Design review of the part built by this model. Coordinates are the model's own, in mm. Face numbers are marked on the shaded views. A direction names the side the tool comes from. Round coordinates to 2 decimals unless told otherwise and drop trailing zeros. Order: outer loops, then holes, each group sorted by start corner. A loop starts at its lowest first (then second) coordinate and runs counter-clockwise, first axis right, second up. Notation, with made-up numbers: M 46.25,88.5 L 91.25,88.5 A23 cw 91.25,98.5 Z; hole C 73,-36 d10. An arc over 180 degrees is marked long. Use a Markdown table: item, result. Add a question column.
(1) Take a section at D-D (x = -9). Write out the cut boundary in (y, z).
(2) Take a section at B-B (z = 2.5). Write out the cut boundary in (x, y), then the cut area to 3 significant figures.
(3) To check wall thickness, follow probe 1 along Z at (x, y) = (10.5, 10); probe 2 along Y at (x, z) = (0, -2.8); probe 3 along Y at (x, z) = (0, -11). State the ranges of each line that lie inside material, in increasing order. Write a range as from..to.
(4) Machinability: for the marked faces 5, 6 and 7, which of the approach directions +Z, -Z, +X, -X, +Y, -Y give a long, thin tool a straight path to every point of the face, cutting with its end or side? Answer none if there is none.
(5) For pin 1 (12 mm diameter, centred on x = 3.5, z = 5, fed in from +Y); pin 2 (3.5 mm diameter, centred on x = -3, y = 1, fed in from +Z); pin 3 (1.5 mm diameter, centred on y = 12, z = -3.5, fed in from -X), all flat-tipped, find the tip position at first contact; note any pin that passes through.
(6) The part is to be moulded in two halves that separate along X. For the marked faces 1, 2, 3 and 4, say which applies: released by +X, released by -X, zero draft, split by the parting line, or undercut.
(7) Take a section at C-C (y = -8.5). Write out the cut boundary in (x, z).
(8) Take a section at A-A (x = 0). Write out the cut boundary in (y, z).
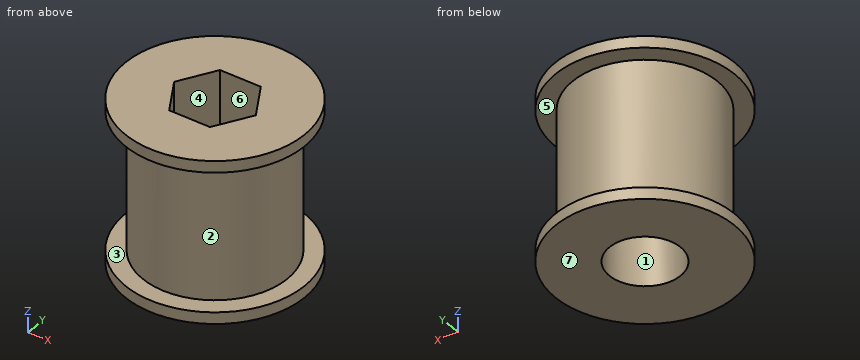
```python
from build123d import *

# Parameters (mm, degrees)
SKETCH1_R           = 12.5
BOSS_EXTRUDE1_DEPTH = 12
SKETCH2_R           = 15.5
BOSS_EXTRUDE2_DEPTH = 2
CUT_EXTRUDE1_DEPTH  = 14
SKETCH5_R           = 2.2
CUT_EXTRUDE2_DEPTH  = 14
SKETCH6_R           = 6.15
CUT_EXTRUDE3_DEPTH  = 10


with BuildPart() as part:
    # Sketch1 → Boss-Extrude1 (new body)
    with BuildSketch(Plane.XY):
        Circle(SKETCH1_R)
    boss_extrude1 = extrude(amount=BOSS_EXTRUDE1_DEPTH)

    # Sketch2 → Boss-Extrude2 (add)
    with BuildSketch(Plane(origin=(0, 0, 12), x_dir=(-1, 0, 0), z_dir=(0, 0, -1))):
        Circle(SKETCH2_R)
    boss_extrude2 = extrude(amount=-BOSS_EXTRUDE2_DEPTH)

    # Sketch3 → Cut-Extrude1 (cut)
    with BuildSketch(Plane.XY):
        Polygon((3.550704156, -6.15), (7.101408311, 0), (3.550704156, 6.15), (-3.550704156, 6.15), (-7.101408311, 0), (-3.550704156, -6.15), align=None)
    extrude(amount=CUT_EXTRUDE1_DEPTH, mode=Mode.SUBTRACT)

    # Mirror1: Boss-Extrude1, Boss-Extrude2 across plane
    add(boss_extrude1.mirror(Plane.XY))
    add(boss_extrude2.mirror(Plane.XY))

    # Sketch5 → Cut-Extrude2 (cut)
    with BuildSketch(Plane.XY):
        Circle(SKETCH5_R)
    extrude(amount=-CUT_EXTRUDE2_DEPTH, mode=Mode.SUBTRACT)

    # Sketch6 → Cut-Extrude3 (cut)
    with BuildSketch(Plane(origin=(0, 0, -14), x_dir=(-1, 0, 0), z_dir=(0, 0, -1))):
        Circle(SKETCH6_R)
    extrude(amount=-CUT_EXTRUDE3_DEPTH, mode=Mode.SUBTRACT)


solid = part.part
```
Verdict:
| question | item | result |
|---|---|---|
| 1 | outline | M -12.62,-14 L 12.62,-14 L 12.62,-12 L 8.67,-12 L 8.67,12 L 12.62,12 L 12.62,14 L -12.62,14 L -12.62,12 L -8.67,12 L -8.67,-12 L -12.62,-12 Z |
| 2 | outline | C 0,0 d25; hole M -7.1,0 L -3.55,-6.15 L 3.55,-6.15 L 7.1,0 L 3.55,6.15 L -3.55,6.15 Z |
| 2 | area | 360 mm^2 |
| 3 | probe 1 | z = -14..-12, 12..14 |
| 3 | probe 2 | y = -12.5..-2.2, 2.2..12.5 |
| 3 | probe 3 | y = -12.5..-6.15, 6.15..12.5 |
| 4 | face 5 | none |
| 4 | face 6 | +Z |
| 4 | face 7 | -Z, +X, -X, +Y, -Y |
| 5 | pin 1 | stops at y = 12.5 |
| 5 | pin 2 | stops at z = 0 |
| 5 | pin 3 | stops at x = -5.45 |
| 6 | face 1 | undercut |
| 6 | face 2 | split by the parting line |
| 6 | face 3 | zero draft |
| 6 | face 4 | undercut |
| 7 | outline | M -12.96,-14 L 12.96,-14 L 12.96,-12 L 9.17,-12 L 9.17,12 L 12.96,12 L 12.96,14 L -12.96,14 L -12.96,12 L -9.17,12 L -9.17,-12 L -12.96,-12 Z |
| 8 | outline | M -15.5,-14 L -6.15,-14 L -6.15,-4 L -2.2,-4 L -2.2,0 L -6.15,0 L -6.15,14 L -15.5,14 L -15.5,12 L -12.5,12 L -12.5,-12 L -15.5,-12 Z; M 2.2,-4 L 6.15,-4 L 6.15,-14 L 15.5,-14 L 15.5,-12 L 12.5,-12 L 12.5,12 L 15.5,12 L 15.5,14 L 6.15,14 L 6.15,0 L 2.2,0 Z |
